For this review, take the finished solid that the model builds, in its own axes (mm). A direction names the side the tool comes from. Coordinates: 2 decimals unless noted, no trailing zeros. Order: outer loops, then holes, each group sorted by start corner. A loop starts at its lowest first (then second) coordinate and runs counter-clockwise, first axis right, second up. Notation, with made-up numbers: M -9,88 L 10,88 A24 cw 10,98 Z; hole C 20.25,81.5 d2. An arc over 180 degrees is marked long. Use one line per item in the form item = value. Start each with the question number.
```python
from build123d import *

# Parameters (mm, degrees)
SKETCH1_R           = 0.254
SKETCH1_W           = 12.7
SKETCH1_H           = 3.4036
SKETCH1_W_2         = 40.386
SKETCH1_H_2         = 19.558
BOSS_EXTRUDE1_DEPTH = 6.35


with BuildPart() as part:
    # Sketch1 → Boss-Extrude1 (new body)
    with BuildSketch(Plane.XY):
        with BuildLine():
            Line((6728.635399657, 3585.149709448), (6728.635399657, 3545.54033771))
            Line((6728.635399657, 3545.54033771), (6735.620399657, 3545.54033771))
            ThreePointArc((6735.620399657, 3545.54033771), (6737.865463687, 3544.61040174), (6738.795399657, 3542.36533771))
            Line((6738.795399657, 3542.36533771), (6738.795399657, 3532.84033771))
            ThreePointArc((6738.795399657, 3532.84033771), (6737.865463687, 3530.595273679), (6735.620399657, 3529.66533771))
            Line((6735.620399657, 3529.66533771), (6728.635399657, 3529.66533771))
            Line((6728.635399657, 3529.66533771), (6728.635399657, 3503.09693771))
            ThreePointArc((6728.635399657, 3503.09693771), (6730.108418233, 3499.540756286), (6733.664599657, 3498.06773771))
            Line((6733.664599657, 3498.06773771), (6733.664599657, 3501.47133771))
            Line((6733.664599657, 3501.47133771), (6746.364599657, 3501.47133771))
            Line((6746.364599657, 3501.47133771), (6746.364599657, 3498.06773771))
            Line((6746.364599657, 3498.06773771), (6791.932199657, 3498.06773771))
            Line((6791.932199657, 3498.06773771), (6791.932199657, 3501.47133771))
            Line((6791.932199657, 3501.47133771), (6804.632199657, 3501.47133771))
            Line((6804.632199657, 3501.47133771), (6804.632199657, 3498.06773771))
            ThreePointArc((6804.632199657, 3498.06773771), (6808.188381081, 3499.540756286), (6809.661399657, 3503.09693771))
            Line((6809.661399657, 3503.09693771), (6809.661399657, 3529.66533771))
            Line((6809.661399657, 3529.66533771), (6802.676399657, 3529.66533771))
            ThreePointArc((6802.676399657, 3529.66533771), (6800.431335626, 3530.595273679), (6799.501399657, 3532.84033771))
            Line((6799.501399657, 3532.84033771), (6799.501399657, 3542.36533771))
            ThreePointArc((6799.501399657, 3542.36533771), (6800.431335626, 3544.61040174), (6802.676399657, 3545.54033771))
            Line((6802.676399657, 3545.54033771), (6809.661399657, 3545.54033771))
            Line((6809.661399657, 3545.54033771), (6809.661399657, 3585.149709448))
            ThreePointArc((6809.661399657, 3585.149709448), (6808.188381081, 3588.705890872), (6804.632199657, 3590.178909448))
            Line((6804.632199657, 3590.178909448), (6804.632199657, 3586.775309448))
            Line((6804.632199657, 3586.775309448), (6791.932199657, 3586.775309448))
            Line((6791.932199657, 3586.775309448), (6791.932199657, 3590.178909448))
            Line((6791.932199657, 3590.178909448), (6746.364599657, 3590.178909448))
            Line((6746.364599657, 3590.178909448), (6746.364599657, 3586.775309448))
            Line((6746.364599657, 3586.775309448), (6733.664599657, 3586.775309448))
            Line((6733.664599657, 3586.775309448), (6733.664599657, 3590.178909448))
            ThreePointArc((6733.664599657, 3590.178909448), (6730.108418233, 3588.705890872), (6728.635399657, 3585.149709448))
        make_face()
        with Locations((6794.416327778, 3547.648139787)):
            Circle(SKETCH1_R, mode=Mode.SUBTRACT)
        with Locations((6794.416327778, 3537.488139787)):
            Circle(SKETCH1_R, mode=Mode.SUBTRACT)
        with Locations((6746.156327778, 3547.648139787)):
            Circle(SKETCH1_R, mode=Mode.SUBTRACT)
        with Locations((6746.156327778, 3537.488139787)):
            Circle(SKETCH1_R, mode=Mode.SUBTRACT)
        with Locations((6748.193399657, 3511.52973771)):
            Rectangle(SKETCH1_W, SKETCH1_H, mode=Mode.SUBTRACT)
        with Locations((6790.103399657, 3511.52973771)):
            Rectangle(SKETCH1_W, SKETCH1_H, mode=Mode.SUBTRACT)
        with Locations((6790.103399657, 3572.79453771)):
            Rectangle(SKETCH1_W, SKETCH1_H, mode=Mode.SUBTRACT)
        with Locations((6748.193399657, 3572.79453771)):
            Rectangle(SKETCH1_W, SKETCH1_H, mode=Mode.SUBTRACT)
        with Locations((6770.286327778, 3542.568139787)):
            Rectangle(SKETCH1_W_2, SKETCH1_H_2, mode=Mode.SUBTRACT)
    extrude(amount=BOSS_EXTRUDE1_DEPTH)


solid = part.part
```
1. Consider section A-A, the plane y = 3550. Write out the cut boundary in (x, z), plus the area to 3 significant figures.
2. To check wall thickness, follow line 1 (Y direction, x = 6792.5, z = 5.5); line 2 (X direction, y = 3510, z = 2.25); line 3 (Y direction, x = 6791, z = 2). State the ranges of each line that lie inside material, in increasing order.
3. For pin 1 Ø1.5 at (x, z) = (6741.5, 2.5) entering from -Y; pin 2 Ø12 at (x, y) = (6774.5, 3534.5) entering from -Z; pin 3 Ø1 at (y, z) = (3588, 4) entering from -X; pin 4 Ø1.7 at (y, z) = (3499.5, 4) entering from +X, all flat-tipped, find the tip position at first contact; note any pin that passes through.
4. Consider section C-C, the plane z = 1.5. Give the number of separate pieces and of enclosed holes in the cut face, plus the area to 3 significant figures.
5. Tool access review of faces 1 (the flat face through (6770, 3552.347, 3)), 2 (the flat face through (6740, 3501.471, 3)), 3 (the cylindrical face through (6730.1, 3588.7, 3.1)), 4 (the cylindrical face through (6800.41, 3544.59, 3.13)), 5 (the flat face through (6769, 3555, 0)): name each direction out of +Z, -Z, +X, -X, +Y, -Y from which nothing blocks a thin tool from reaching the whole face with its end or side.
6. Consider section B-B, the plane x = 6767. Write out the cut boundary in (y, z), plus the area to 3 significant figures.
7. The part is to be moulded in two halves that separate along Y. For faces 6 (the flat face through (6769, 3590.179, 3)), 7 (the flat face through (6748, 3509.828, 3)), 8 (the flat face through (6746.365, 3500, 3)), say which applies: pulls with the +Y half, pulls with the -Y half, needs draft (parallel to the pull), parting line crosses it, or undercut.
Answers follow:
q1.outline = M 6728.64,0 L 6750.09,0 L 6750.09,6.35 L 6728.64,6.35 Z; M 6790.48,0 L 6809.66,0 L 6809.66,6.35 L 6790.48,6.35 Z
q1.area = 258 mm²
q2.line_1 = 3501.47 to 3509.83, 3513.23 to 3571.09, 3574.5 to 3586.78
q2.line_2 = 6728.64 to 6741.84, 6754.54 to 6783.75, 6796.45 to 6809.66
q2.line_3 = 3498.07 to 3509.83, 3513.23 to 3571.09, 3574.5 to 3590.18
q3.pin_1 = 3501.47
q3.pin_2 = 0
q3.pin_3 = 6729.22
q3.pin_4 = 6808.84
q4.separate_pieces = 1
q4.enclosed_holes = 9
q4.area = 5,990 mm²
q5.face_1 = +Z, -Z
q5.face_2 = +Z, -Z, -Y
q5.face_3 = +Z, -Z, -X, +Y
q5.face_4 = +Z, -Z, +X
q5.face_5 = -Z, +X, -X, +Y, -Y
q6.outline = M 3498.07,0 L 3532.79,0 L 3532.79,6.35 L 3498.07,6.35 Z; M 3552.35,0 L 3590.18,0 L 3590.18,6.35 L 3552.35,6.35 Z
q6.area = 461 mm²
q7.face_6 = pulls with the +Y half
q7.face_7 = undercut
q7.face_8 = needs draft
